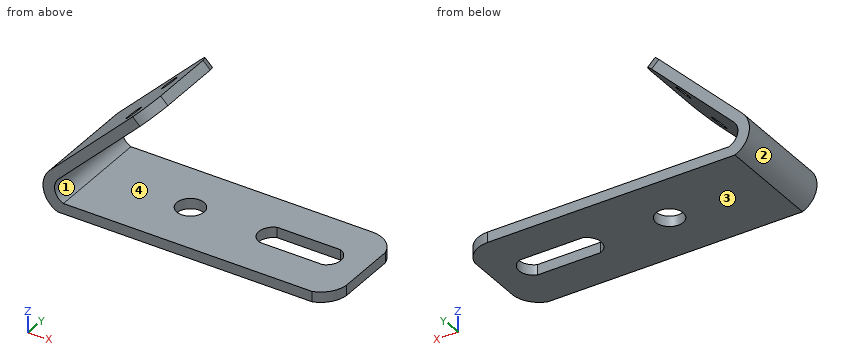
from build123d import *

# Parameters (mm, degrees)
F1_DEPTH = 483.87
F2_R     = 63.5
F2_W     = 292.9965630609
F2_H     = 127
F3_DEPTH = 48.261
F4_R     = 38.1
F5_DEPTH = 78.74
F6_DEPTH = 483.871


with BuildPart() as f1:
    # F0 (on Front) → F1 (new body)
    with BuildSketch(Plane.XZ):
        with BuildLine():
            Line((769.3116354294, -399.2148596497), (769.3116354294, -350.9548596497))
            Line((769.3116354294, -350.9548596497), (-473.3476042747, -350.9548596497))
            ThreePointArc((-473.3476042747, -350.9548596497), (-513.072288863, -303.7029004261), (-495.3859384083, -244.5590822901))
            Line((-495.3859384083, -244.5590822901), (-46.3731323549, 204.4537237633))
            Line((-46.3731323549, 204.4537237633), (-86.3926232658, 231.4253374939))
            Line((-86.3926232658, 231.4253374939), (-535.4054293192, -217.5874685596))
            ThreePointArc((-535.4054293192, -217.5874685596), (-566.1518276604, -317.596153827), (-500.6883645706, -399.2148596497))
            Line((-500.6883645706, -399.2148596497), (769.3116354294, -399.2148596497))
        make_face()
    extrude(amount=-F1_DEPTH)

    # F2 (on face) → F3 (cut, through all)
    with BuildSketch(Plane.XY.offset(-350.9548596497)):
        with Locations((-43.4883645706, 246.7185220676)):
            Circle(F2_R)
        with Locations((464.5116354294, 246.7185220676)):
            Rectangle(F2_W, F2_H)
        with BuildLine():
            ThreePointArc((611.0099169598, 183.2185220676), (655.0116354294, 246.7185220676), (611.0099169598, 310.2185220676))
            Line((611.0099169598, 310.2185220676), (611.0099169598, 183.2185220676))
        make_face()
        with BuildLine():
            Line((318.013353899, 183.2185220676), (318.013353899, 310.2185220676))
            ThreePointArc((318.013353899, 310.2185220676), (274.0116354294, 246.7185220676), (318.013353899, 183.2185220676))
        make_face()
        with BuildLine():
            ThreePointArc((647.7836660054, 483.87), (724.587147216, 456.9907780756), (769.3116354294, 389.0129327774))
            Line((769.3116354294, 389.0129327774), (769.3116354294, 483.87))
            Line((769.3116354294, 483.87), (647.7836660054, 483.87))
        make_face()
        with BuildLine():
            Line((769.3116354294, 0), (769.3116354294, 110.9018325806))
            ThreePointArc((769.3116354294, 110.9018325806), (742.030303117, 41.9598138448), (680.9021830559, 0))
            Line((680.9021830559, 0), (769.3116354294, 0))
        make_face()
    extrude(amount=-F3_DEPTH, mode=Mode.SUBTRACT)

    # F4 (on face) → F5 (cut)
    with BuildSketch(Plane(origin=(-158.9089803798, 0, 158.9089803798), x_dir=(0, -1, 0), z_dir=(-0.7071067812, 0, 0.7071067812))):
        with Locations((-369.57, -87.9463842754)):
            Circle(F4_R)
        with Locations((-114.3, -87.9463842754)):
            Circle(F4_R)
        with BuildLine():
            ThreePointArc((-99.5377227664, 102.5536157246), (-36.434263942, 70.8775530516), (0, 10.3964496136))
            Line((0, 10.3964496136), (0, 102.5536157246))
            Line((0, 102.5536157246), (-99.5377227664, 102.5536157246))
        make_face()
        with BuildLine():
            ThreePointArc((-483.87, 16.0886850208), (-454.0610525131, 69.3496689518), (-402.8477370739, 102.5536157246))
            Line((-402.8477370739, 102.5536157246), (-483.87, 102.5536157246))
            Line((-483.87, 102.5536157246), (-483.87, 16.0886850208))
        make_face()
    extrude(amount=-F5_DEPTH, mode=Mode.SUBTRACT)

    # F6 (cut, through all): a face of the model
    f6_faces = [f1.faces().sort_by_distance(p)[0] for p in [
        (-61.8876088552, 0, 211.2696154768),
    ]]
    extrude(f6_faces, amount=-F6_DEPTH, mode=Mode.SUBTRACT)


solid = f1.part
Geometry check sheet. Reference: the model listing, model coordinates, mm. Face numbers are marked on the shaded views. Round coordinates to 2 decimals unless told otherwise and drop trailing zeros. Order: outer loops, then holes, each group sorted by start corner. A loop starts at its lowest first (then second) coordinate and runs counter-clockwise, first axis right, second up. Notation, with made-up numbers: M 81.5,-16.75 L 99.5,-16.75 A10 ccw 99.5,2.25 Z; hole C 57.25,22.25 d11. An arc over 180 degrees is marked long. Answer in a Markdown table with one row per item. Add a question column.
Item 1: Sectioned sample at D-D, the plane x = 141.5. Enter the section's corners in (y, z).
Item 2: Sectioned sample at B-B, the plane x = -31. Enter the section's corners in (y, z).
Item 3: Depth check by flat-ended pin: pin 1 Ø1.5 at (x, y) = (627, 386.5) entering from +Z; pin 2 Ø8 at (y, z) = (78.5, -192) entering from +X; pin 3 Ø4 at (y, z) = (280, -227) entering from +X. Enter the tip coordinate at first touch or a pass-through.
Item 4: Draft check along Z on the marked faces 1, 2, 3 and 4. Enter one of: released by +Z, released by -Z, zero draft, split by the parting line, or undercut.
Item 5: Material ranges on L1, parallel to Z at x = 95.5, y = 89; L2, parallel to Z at x = -339.5, y = 436.5; L3, parallel to Z at x = -279.5, y = 73.5, recorded low to high. Write a range as [from, to].
Item 6: Sectioned sample at A-A, the plane y = 202. Enter the section's corners in (x, z).
Item 7: Sectioned sample at C-C, the plane y = 451. Enter the section's corners in (x, z).
Filled in:
| question | item | result |
|---|---|---|
| 1 | outline | M 0,-399.21 L 483.87,-399.21 L 483.87,-350.95 L 0,-350.95 Z |
| 2 | outline | M 0,-399.21 L 184.46,-399.21 L 184.46,-350.95 L 0,-350.95 Z; M 308.98,-399.21 L 483.87,-399.21 L 483.87,-350.95 L 308.98,-350.95 Z |
| 3 | pin 1 | stops at z = -350.95 |
| 3 | pin 2 | stops at x = -438.83 |
| 3 | pin 3 | stops at x = -475.83 |
| 4 | face 1 | undercut |
| 4 | face 2 | split by the parting line |
| 4 | face 3 | released by -Z |
| 4 | face 4 | undercut |
| 5 | L1 | z = [-399.21, -350.95] |
| 5 | L2 | z = [-399.21, -350.95], [-88.67, -21.68] |
| 5 | L3 | z = [-399.21, -350.95], [-28.67, 38.32] |
| 6 | outline | M -535.41,-217.59 A111.76 ccw -500.69,-399.21 L -88.57,-399.21 L -88.57,-350.95 L -473.35,-350.95 A65 cw -495.39,-244.56 L -52.9,197.93 L -86.39,231.43 Z; M 1.59,-399.21 L 290.84,-399.21 L 290.84,-350.95 L 1.59,-350.95 Z; M 638.18,-399.21 L 769.31,-399.21 L 769.31,-350.95 L 638.18,-350.95 Z |
| 7 | outline | M -535.41,-217.59 A111.76 ccw -500.69,-399.21 L 731.71,-399.21 L 731.71,-350.95 L -473.35,-350.95 A65 cw -495.39,-244.56 L -74.14,176.68 L -107.64,210.18 Z |
